from build123d import *

# Parameters (mm, degrees)
F0_R     = 9.5
F0_R_2   = 8.5
F1_DEPTH = 3.5
F0_R_3   = 8.25
F0_R_4   = 7.25
F2_DEPTH = 1
F3_DEPTH = 2


with BuildPart() as f1:
    # F0 (on Top) → F1 (new body)
    with BuildSketch(Plane.XY):
        Circle(F0_R)
        Circle(F0_R_2, mode=Mode.SUBTRACT)
    extrude(amount=F1_DEPTH)

    # F0 (on Top) → F2 (join)
    with BuildSketch(Plane.XY):
        Circle(F0_R)
        Circle(F0_R_2, mode=Mode.SUBTRACT)
        Circle(F0_R_2)
        Circle(F0_R_3, mode=Mode.SUBTRACT)
        Circle(F0_R_3)
        Circle(F0_R_4, mode=Mode.SUBTRACT)
        Circle(F0_R_4)
    extrude(amount=-F2_DEPTH)

    # F0 (on Top) → F3 (join)
    with BuildSketch(Plane.XY):
        Circle(F0_R_3)
        Circle(F0_R_4, mode=Mode.SUBTRACT)
    extrude(amount=-F3_DEPTH)


solid = f1.part
Source: CAD feature listing. Evaluate the final solid. Frame: model axes, mm. A direction names the side the tool comes from. Round coordinates to 2 decimals unless told otherwise and drop trailing zeros. Loops run counter-clockwise (first coordinate to the right, second up) from the corner with the lowest first, then second, coordinate; pieces in that order, holes last. Notation, with made-up numbers: M 48.25,78 L 106.25,78 A26 cw 106.25,117 Z; hole C 52.5,-25 d11. An arc over 180 degrees is marked long. Answer as CSV lines item,"result".
Q1. Cut plane A-A (x = 0). Return the cut outline in (y, z).
Verdict:
outline,"M -9.5,-1 L -8.25,-1 L -8.25,-2 L -7.25,-2 L -7.25,-1 L 7.25,-1 L 7.25,-2 L 8.25,-2 L 8.25,-1 L 9.5,-1 L 9.5,3.5 L 8.5,3.5 L 8.5,0 L -8.5,0 L -8.5,3.5 L -9.5,3.5 Z"
Q2. Pull-direction query (X, two-part tool) for faces 4 (the face through (-2.2, -8.4, 3.5)), 5 (the face through (4.38, -8.43, 1.28)), 6 (the face through (3.35, -6.43, -1.49)); classes: +X half, -X half, draft (parallel to the pull), parting line (faces both ways), or undercut.
Verdict:
face 4,"draft"
face 5,"parting line"
face 6,"undercut"
Q3. Line query: line 1 along Y through (x, z) = (0, -1.7); line 2 along Y through (x, z) = (0, 2.6); line 3 along Z through (x, y) = (-7.5, 0.75). Output: solid intervals per line, ascending.
Verdict:
line 1,"y = -8.25 to -7.25, 7.25 to 8.25"
line 2,"y = -9.5 to -8.5, 8.5 to 9.5"
line 3,"z = -2 to 0"
Q4. Contact query for flat-ended pins moving along their axis: pin 1 (3 mm diameter, centred on x = 3, z = 1.5, fed in from +Y); pin 2 (1 mm diameter, centred on x = 1, y = 1, fed in from +Z); pin 3 (7 mm diameter, centred on x = 0, y = 2, fed in from -Z). Output: stop coordinate, or through.
Verdict:
pin 1,"stops at y = 9.38"
pin 2,"stops at z = 0"
pin 3,"stops at z = -1"
Q5. Reachability of faces 1 (the face through (4.57, 7.167, 1.726)), 2 (the face through (3, -7, -2)), 3 (the face through (0, 0, -1)) from +Z, -Z, +X, -X, +Y, -Y: full face, straight path, thin tool, end or side. Return the list, or none.
Verdict:
face 1,"+Z"
face 2,"-Z, +X, -X, +Y, -Y"
face 3,"-Z"
Q6. Cut plane C-C (z = -1.55). Return the cut outline in (x, y).
Verdict:
outline,"C 0,0 d16.5; hole C 0,0 d14.5"
Q7. Cut plane D-D (y = -7.5). Return the cut outline in (x, z).
Verdict:
outline,"M -5.83,-1 L -3.44,-1 L -3.44,-2 L 3.44,-2 L 3.44,-1 L 5.83,-1 L 5.83,3.5 L 4,3.5 L 4,0 L -4,0 L -4,3.5 L -5.83,3.5 Z"
